from build123d import *

# Parameters (mm, degrees)
SKETCH_1_W          = 155
SKETCH_1_H          = 28
EXTRUDE_1_DEPTH     = 3
CUT_EXTRUDE_1_REACH = 80.811
SKETCH_2_R          = 4.25
SKETCH_2_R_2        = 2.25
FILLET_1_RADIUS     = 14
FILLET_1_LENGTH     = 3
CUT_EXTRUDE_2_REACH = 80.811
SKETCH_3_R          = 2.25
FILLET_2_RADIUS     = 14
FILLET_2_LENGTH     = 3


with BuildPart() as part:
    # 草图1 → 凸台-拉伸1 (new body)
    with BuildSketch(Plane(origin=(0, 0, 0), x_dir=(1, 0, 0), z_dir=(0, 1, 0))):
        Rectangle(SKETCH_1_W, SKETCH_1_H)
    extrude(amount=EXTRUDE_1_DEPTH)

    # 草图2 → 切除-拉伸1 (cut, up to next)
    with BuildSketch(Plane(origin=(0, 3, 0), x_dir=(1, 0, 0), z_dir=(0, 1, 0)), mode=Mode.PRIVATE) as cut_extrude_1_sk1:
        with Locations(Location((-50, 0, 0), (0, 0, 270))):
            Circle(SKETCH_2_R)
    cut_extrude_1_tool1 = extrude(cut_extrude_1_sk1.sketch, amount=-CUT_EXTRUDE_1_REACH, mode=Mode.PRIVATE) & part.part
    # 草图2 → 切除-拉伸1 (cut, up to next)
    with BuildSketch(Plane(origin=(0, 3, 0), x_dir=(1, 0, 0), z_dir=(0, 1, 0)), mode=Mode.PRIVATE) as cut_extrude_1_sk2:
        with Locations(Location((50, 0, 0), (0, 0, 270))):
            Circle(SKETCH_2_R)
    cut_extrude_1_tool2 = extrude(cut_extrude_1_sk2.sketch, amount=-CUT_EXTRUDE_1_REACH, mode=Mode.PRIVATE) & part.part
    # 草图2 → 切除-拉伸1 (cut, up to next)
    with BuildSketch(Plane(origin=(0, 3, 0), x_dir=(1, 0, 0), z_dir=(0, 1, 0)), mode=Mode.PRIVATE) as cut_extrude_1_sk3:
        with Locations(Location((0, 0, 0), (0, 0, 270))):
            Circle(SKETCH_2_R_2)
    cut_extrude_1_tool3 = extrude(cut_extrude_1_sk3.sketch, amount=-CUT_EXTRUDE_1_REACH, mode=Mode.PRIVATE) & part.part
    add(cut_extrude_1_tool1.solids().sort_by_distance((-50, 3, 0))[0], mode=Mode.SUBTRACT)
    add(cut_extrude_1_tool2.solids().sort_by_distance((50, 3, 0))[0], mode=Mode.SUBTRACT)
    add(cut_extrude_1_tool3.solids().sort_by_distance((0, 3, 0))[0], mode=Mode.SUBTRACT)

    # 圆角1: full round fillet: the end face becomes a half cylinder, R = half its width
    fillet_1_face = Plane((-77.5, 1.5, 0), x_dir=(0, 1, 0), z_dir=(-1, 0, 0))  # on the end face: x along it, z out of the body
    fillet_1_slab = fillet_1_face.offset(-FILLET_1_RADIUS / 2) * Box(FILLET_1_LENGTH, 2 * FILLET_1_RADIUS, FILLET_1_RADIUS, mode=Mode.PRIVATE)  # the body's end, R deep
    fillet_1_round = Plane((-63.5, 1.5, 0), x_dir=(-1, 0, 0), z_dir=(0, 1, 0)) * Cylinder(FILLET_1_RADIUS, FILLET_1_LENGTH, mode=Mode.PRIVATE)  # its axis R under the face
    add(fillet_1_slab - fillet_1_round, mode=Mode.SUBTRACT)

    # 草图3 → 切除-拉伸2 (cut, up to next)
    with BuildSketch(Plane(origin=(0, 3, 0), x_dir=(1, 0, 0), z_dir=(0, 1, 0)), mode=Mode.PRIVATE) as cut_extrude_2_sk1:
        with Locations(Location((-68.5, 0, 0), (0, 0, 270))):
            Circle(SKETCH_3_R)
    cut_extrude_2_tool1 = extrude(cut_extrude_2_sk1.sketch, amount=-CUT_EXTRUDE_2_REACH, mode=Mode.PRIVATE) & part.part
    # 草图3 → 切除-拉伸2 (cut, up to next)
    with BuildSketch(Plane(origin=(0, 3, 0), x_dir=(1, 0, 0), z_dir=(0, 1, 0)), mode=Mode.PRIVATE) as cut_extrude_2_sk2:
        with Locations(Location((-31.5, 0, 0), (0, 0, 270))):
            Circle(SKETCH_3_R)
    cut_extrude_2_tool2 = extrude(cut_extrude_2_sk2.sketch, amount=-CUT_EXTRUDE_2_REACH, mode=Mode.PRIVATE) & part.part
    # 草图3 → 切除-拉伸2 (cut, up to next)
    with BuildSketch(Plane(origin=(0, 3, 0), x_dir=(1, 0, 0), z_dir=(0, 1, 0)), mode=Mode.PRIVATE) as cut_extrude_2_sk3:
        with Locations(Location((31.5, 0, 0), (0, 0, 270))):
            Circle(SKETCH_3_R)
    cut_extrude_2_tool3 = extrude(cut_extrude_2_sk3.sketch, amount=-CUT_EXTRUDE_2_REACH, mode=Mode.PRIVATE) & part.part
    # 草图3 → 切除-拉伸2 (cut, up to next)
    with BuildSketch(Plane(origin=(0, 3, 0), x_dir=(1, 0, 0), z_dir=(0, 1, 0)), mode=Mode.PRIVATE) as cut_extrude_2_sk4:
        with Locations(Location((68.5, 0, 0), (0, 0, 270))):
            Circle(SKETCH_3_R)
    cut_extrude_2_tool4 = extrude(cut_extrude_2_sk4.sketch, amount=-CUT_EXTRUDE_2_REACH, mode=Mode.PRIVATE) & part.part
    add(cut_extrude_2_tool1.solids().sort_by_distance((-68.5, 3, 0))[0], mode=Mode.SUBTRACT)
    add(cut_extrude_2_tool2.solids().sort_by_distance((-31.5, 3, 0))[0], mode=Mode.SUBTRACT)
    add(cut_extrude_2_tool3.solids().sort_by_distance((31.5, 3, 0))[0], mode=Mode.SUBTRACT)
    add(cut_extrude_2_tool4.solids().sort_by_distance((68.5, 3, 0))[0], mode=Mode.SUBTRACT)

    # 圆角2: full round fillet: the end face becomes a half cylinder, R = half its width
    fillet_2_face = Plane((77.5, 1.5, 0), x_dir=(0, -1, 0), z_dir=(1, 0, 0))  # on the end face: x along it, z out of the body
    fillet_2_slab = fillet_2_face.offset(-FILLET_2_RADIUS / 2) * Box(FILLET_2_LENGTH, 2 * FILLET_2_RADIUS, FILLET_2_RADIUS, mode=Mode.PRIVATE)  # the body's end, R deep
    fillet_2_round = Plane((63.5, 1.5, 0), x_dir=(1, 0, 0), z_dir=(0, -1, 0)) * Cylinder(FILLET_2_RADIUS, FILLET_2_LENGTH, mode=Mode.PRIVATE)  # its axis R under the face
    add(fillet_2_slab - fillet_2_round, mode=Mode.SUBTRACT)


solid = part.part
Design review of the part built by this model. Coordinates are the model's own, in mm. Round coordinates to 2 decimals unless told otherwise and drop trailing zeros. Write each loop counter-clockwise with the first axis right and the second up, starting at its lowest first coordinate (ties: lowest second). Pieces come first, ordered by that corner, then holes.
Item 1: Draft analysis for pull direction X (two halves, no side actions). For faces 1 (the flat face through (-1, 0, 3)), 2 (the cylindrical face through (-77.497, 1.521, -0.308)), 3 (the cylindrical face through (-32.869, 1.521, -1.786)), state which applies: released by +X, released by -X, zero draft, split by the parting line, or undercut.
Item 2: Consider section C-C on y = 2.3. Give the boundary of the cut face in (x, z).
Item 3: Consider section A-A on x = 31.5. Give the boundary of the cut face in (y, z).
Item 4: Consider section D-D on x = -50. Give the boundary of the cut face in (y, z).
Item 5: Consider section B-B on z = 0. Count the separate pieces of the cut face and the enclosed holes in it, and give its area (4 significant figures).
Item 6: Wall thickness on L1, parallel to X at y = 2.25, z = 2.5; L2, parallel to Z at x = -32, y = 2.1; L3, parallel to X at y = 2.25, z = 9.5: over which ranges is each line inside the solid? List them lowest first.
Check values:
1. face 1: zero draft
1. face 2: released by -X
1. face 3: undercut
2. outline: (-63.5, -14) - (63.5, -14) arc R14 ccw to (63.5, 14) - (-63.5, 14) arc R14 ccw to start; hole circle Ø4.5 at (-68.5, 0); hole circle Ø8.5 at (-50, 0); hole circle Ø4.5 at (-31.5, 0); hole circle Ø4.5 at (0, 0); hole circle Ø4.5 at (31.5, 0); hole circle Ø8.5 at (50, 0); hole circle Ø4.5 at (68.5, 0)
3. outline: (0, -14) - (3, -14) - (3, -2.25) - (0, -2.25) - close; (0, 2.25) - (3, 2.25) - (3, 14) - (0, 14) - close
4. outline: (0, -14) - (3, -14) - (3, -4.25) - (0, -4.25) - close; (0, 4.25) - (3, 4.25) - (3, 14) - (0, 14) - close
5. separate pieces: 8
5. enclosed holes: 0
5. area: 346.5 mm2
6. L1: x = -77.27 to -53.44, -46.56 to 46.56, 53.44 to 77.27
6. L2: z = -14 to -2.19, 2.19 to 14
6. L3: x = -73.78 to 73.78
